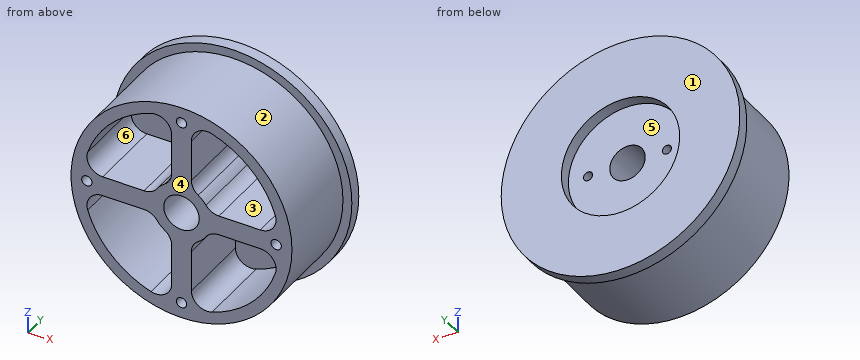
Solid Edge part; units mm, degrees
sketch "Sketch1" plane through (0, 0, 0) normal (0, -1, 0) x (1, 0, 0)
  circle A0 centre (0, 0) radius 30.25
extrude "Protrusion1" add sketch "Sketch1" along normal blind 3
sketch "Sketch2" plane through (0, -3, 0) normal (0, -1, 0) x (1, 0, 0)
  circle A0 centre (0, 0) radius 28
extrude "ExtrudedProtrusion_2" add sketch "Sketch2" along normal blind 22
sketch "Sketch3" plane through (0, 0, 0) normal (0, 1, 0) x (-1, 0, 0)
  circle A0 centre (0, 0) radius 15
extrude "ExtrudedCutout_1" cut sketch "Sketch3" against normal blind 3 and the other way up to next
sketch "Sketch4" plane through (0, -25, 0) normal (0, -1, 0) x (1, 0, 0)
  circle A0 centre (0, 0) radius 4.5
extrude "Cutout1" cut sketch "Sketch4" against normal through all and the other way up to next
sketch "Sketch5" plane through (0, -3, 0) normal (0, 1, 0) x (-1, 0, 0)
  circle A0 centre (-10, 0) radius 1.15
  circle A1 centre (10, 0) radius 1.15
extrude "ExtrudedCutout_3" cut sketch "Sketch5" against normal blind 15 and the other way up to next
sketch "Sketch6" plane through (0, -25, 0) normal (0, -1, 0) x (0, 0, -1)
  arc A0 (-24.8747, 2.5) -> (-2.5, 24.8747) centre (0, 0) cw
  line L0 (-2.5, 7.0711) -> (-2.5, 24.8747)
  arc A1 (-7.0711, 2.5) -> (-2.5, 7.0711) centre (0, 0) cw
  line L1 (-7.0711, 2.5) -> (-24.8747, 2.5)
  line L2 (7.0711, 2.5) -> (24.8747, 2.5)
  line L3 (2.5, 24.8747) -> (2.5, 7.0711)
  arc A2 (2.5, 24.8747) -> (24.8747, 2.5) centre (0, 0) cw
  arc A3 (2.5, 7.0711) -> (7.0711, 2.5) centre (0, 0) cw
  line L4 (7.0711, -2.5) -> (24.8747, -2.5)
  arc A4 (24.8747, -2.5) -> (2.5, -24.8747) centre (0, 0) cw
  line L5 (2.5, -7.0711) -> (2.5, -24.8747)
  arc A5 (7.0711, -2.5) -> (2.5, -7.0711) centre (0, 0) cw
  arc A6 (-2.5, -7.0711) -> (-7.0711, -2.5) centre (0, 0) cw
  line L6 (-7.0711, -2.5) -> (-24.8747, -2.5)
  arc A7 (-2.5, -24.8747) -> (-24.8747, -2.5) centre (0, 0) cw
  line L7 (-2.5, -7.0711) -> (-2.5, -24.8747)
extrude "ExtrudedCutout_4" cut sketch "Sketch6" against normal blind 19 and the other way up to next
fillet "Round_1" radius 4 16 edges at (2.5, -15.5, 24.8747) (-2.5, -15.5, 24.8747) (2.5, -15.5, 7.0711) (7.0711, -15.5, 2.5) (24.8747, -15.5, 2.5) (24.8747, -15.5, -2.5) (7.0711, -15.5, -2.5) (2.5, -15.5, -7.0711) (2.5, -15.5, -24.8747) (-2.5, -15.5, -24.8747) (-2.5, -15.5, -7.0711) (-7.0711, -15.5, -2.5) (-2.5, -15.5, 7.0711) (-7.0711, -15.5, 2.5) (-24.8747, -15.5, 2.5) (-24.8747, -15.5, -2.5)
sketch "Sketch7" plane through (0, -25, 0) normal (0, -1, 0) x (0, 0, -1)
  circle A0 centre (0, 24) radius 1.3
  circle A1 centre (-24, 0) radius 1.3
  circle A2 centre (24, 0) radius 1.3
  circle A3 centre (0, -24) radius 1.3
extrude "ExtrudedCutout_5" cut sketch "Sketch7" against normal blind 20 and the other way up to next
Work out the finished part from the listing and answer in its coordinate system (mm). Face numbers are marked on the shaded views. A direction names the side the tool comes from. Give positions to 0.01 mm unless a question says otherwise; leave off trailing zeros. Loops run counter-clockwise (first coordinate to the right, second up) from the corner with the lowest first, then second, coordinate; pieces in that order, holes last. Notation, with made-up numbers: (1, 26.5) -> (40, 26.5) arc R23 cw to (40, 61.5) -> close; hole circle Ø10 at (-3, 24). An arc over 180 degrees is marked (long way). Use a Markdown table: item, result. Add a question column.
1. Flat-ended cylindrical pins translate along their axes: pin 1 Ø1 at (y, z) = (-17, -1) entering from -X; pin 2 Ø2 at (x, z) = (-24, 0.5) entering from -Y; pin 3 Ø3.5 at (x, z) = (10, 0) entering from +Y; pin 4 Ø10 at (x, y) = (-23, -10) entering from -Z. Find the tip coordinate at first contact, or state that the pin passes through.
2. Find the intervals of material crossed by probe 1 along X at (y, z) = (-4.5, -1); probe 2 along X at (y, z) = (-16.75, -7.5); probe 3 along Z at (x, y) = (-10, -15), in increasing order.
3. Determine the mould class of the marked faces 1, 2 and 3 for opening direction Z: released by +Z, released by -Z, zero draft, split by the parting line, or undercut.
4. Section D-D on x = -12.5 is taken. Determine the outline of the cut face in (y, z), and give its area (3 significant figures).
5. Section B-B on x = 0 is taken. Determine the outline of the cut face in (y, z).
6. Section C-C on y = -2.25 is taken. Determine the outline of the cut face in (x, z).
7. For the marked faces 4, 5 and 6, determine the directions among +Z, -Z, +X, -X, +Y, -Y from which every point of the face is accessible in a straight line to the end or side of a thin tool.
Results below:
| question | item | result |
|---|---|---|
| 1 | pin 1 | stops at x = -28 |
| 1 | pin 2 | stops at y = -25 |
| 1 | pin 3 | stops at y = -3 |
| 1 | pin 4 | stops at z = -21.45 |
| 2 | probe 1 | x = -27.98 to -10.57, -9.43 to -4.39, 4.39 to 9.43, 10.57 to 27.98 |
| 2 | probe 2 | x = -26.98 to -23.84, -3.03 to 3.03, 23.84 to 26.98 |
| 2 | probe 3 | z = -26.15 to -22.91, -2.5 to -1.15, 1.15 to 2.5, 22.91 to 26.15 |
| 3 | face 1 | zero draft |
| 3 | face 2 | split by the parting line |
| 3 | face 3 | undercut |
| 4 | outline | (-25, -25.05) -> (-3, -25.05) -> (-3, -27.55) -> (0, -27.55) -> (0, -8.29) -> (-3, -8.29) -> (-3, 8.29) -> (0, 8.29) -> (0, 27.55) -> (-3, 27.55) -> (-3, 25.05) -> (-25, 25.05) -> (-25, 21.65) -> (-6, 21.65) -> (-6, 2.5) -> (-25, 2.5) -> (-25, -2.5) -> (-6, -2.5) -> (-6, -21.65) -> (-25, -21.65) -> close |
| 4 | area | 490 mm^2 |
| 5 | outline | (-25, -28) -> (-3, -28) -> (-3, -30.25) -> (0, -30.25) -> (0, -15) -> (-3, -15) -> (-3, -4.5) -> (-25, -4.5) -> (-25, -22.7) -> (-5, -22.7) -> (-5, -25.3) -> (-25, -25.3) -> close; (-25, 4.5) -> (-3, 4.5) -> (-3, 15) -> (0, 15) -> (0, 30.25) -> (-3, 30.25) -> (-3, 28) -> (-25, 28) -> (-25, 25.3) -> (-5, 25.3) -> (-5, 22.7) -> (-25, 22.7) -> close |
| 6 | outline | circle Ø60.5 at (0, 0); hole circle Ø30 at (0, 0) |
| 7 | face 4 | +Z, -Z, +X, -X, -Y |
| 7 | face 5 | +Y |
| 7 | face 6 | -Y |
